Geometry: final body of the model. Coordinates: model frame, mm. Give positions to 0.01 mm unless a question says otherwise; leave off trailing zeros. Order: outer loops, then holes, each group sorted by start corner. A loop starts at its lowest first (then second) coordinate and runs counter-clockwise, first axis right, second up. Notation, with made-up numbers: (84.5, -25.75) -> (115.5, -25.75) arc R31 cw to (115.5, 4.25) -> close; hole circle Ø7 at (32, 89). An arc over 180 degrees is marked (long way). One line per item, written item: value. Start each with the question number.
```python
from build123d import *

# Parameters (mm, degrees)
SKETCH1_R           = 85.725
BOSS_EXTRUDE1_DEPTH = 6.35
CUT_EXTRUDE1_REACH  = 123.4
SKETCH2_R           = 1.5875
CUT_EXTRUDE2_REACH  = 123.4
SKETCH3_R           = 5
SKETCH3_R_2         = 3.175
CUT_EXTRUDE3_REACH  = 123.4
SKETCH5_R           = 1.4732
CENTER_HOLE_REACH   = 123.4
SKETCH6_R           = 5.0165


with BuildPart() as part:
    # Sketch1 → Boss-Extrude1 (new body)
    with BuildSketch(Plane(origin=(0, 0, 0), x_dir=(1, 0, 0), z_dir=(0, 1, 0))):
        with Locations(Location((0, 0, 0), (0, 0, 270))):
            Circle(SKETCH1_R)
    extrude(amount=BOSS_EXTRUDE1_DEPTH)

    # Sketch2 → Cut-Extrude1 (cut, up to next)
    with BuildSketch(Plane(origin=(0, 6.35, 0), x_dir=(1, 0, 0), z_dir=(0, 1, 0)), mode=Mode.PRIVATE) as cut_extrude1_sk1:
        with Locations(Location((-63.5, 44.45, 0), (0, 0, 270))):
            Circle(SKETCH2_R)
    cut_extrude1_tool1 = extrude(cut_extrude1_sk1.sketch, amount=-CUT_EXTRUDE1_REACH, mode=Mode.PRIVATE) & part.part
    # Sketch2 → Cut-Extrude1 (cut, up to next)
    with BuildSketch(Plane(origin=(0, 6.35, 0), x_dir=(1, 0, 0), z_dir=(0, 1, 0)), mode=Mode.PRIVATE) as cut_extrude1_sk2:
        with Locations(Location((63.5, 44.45, 0), (0, 0, 270))):
            Circle(SKETCH2_R)
    cut_extrude1_tool2 = extrude(cut_extrude1_sk2.sketch, amount=-CUT_EXTRUDE1_REACH, mode=Mode.PRIVATE) & part.part
    # Sketch2 → Cut-Extrude1 (cut, up to next)
    with BuildSketch(Plane(origin=(0, 6.35, 0), x_dir=(1, 0, 0), z_dir=(0, 1, 0)), mode=Mode.PRIVATE) as cut_extrude1_sk3:
        with Locations(Location((-63.5, -44.45, 0), (0, 0, 270))):
            Circle(SKETCH2_R)
    cut_extrude1_tool3 = extrude(cut_extrude1_sk3.sketch, amount=-CUT_EXTRUDE1_REACH, mode=Mode.PRIVATE) & part.part
    # Sketch2 → Cut-Extrude1 (cut, up to next)
    with BuildSketch(Plane(origin=(0, 6.35, 0), x_dir=(1, 0, 0), z_dir=(0, 1, 0)), mode=Mode.PRIVATE) as cut_extrude1_sk4:
        with Locations(Location((63.5, -44.45, 0), (0, 0, 270))):
            Circle(SKETCH2_R)
    cut_extrude1_tool4 = extrude(cut_extrude1_sk4.sketch, amount=-CUT_EXTRUDE1_REACH, mode=Mode.PRIVATE) & part.part
    add(cut_extrude1_tool1.solids().sort_by_distance((-63.5, 6.35, -44.45))[0], mode=Mode.SUBTRACT)
    add(cut_extrude1_tool2.solids().sort_by_distance((63.5, 6.35, -44.45))[0], mode=Mode.SUBTRACT)
    add(cut_extrude1_tool3.solids().sort_by_distance((-63.5, 6.35, 44.45))[0], mode=Mode.SUBTRACT)
    add(cut_extrude1_tool4.solids().sort_by_distance((63.5, 6.35, 44.45))[0], mode=Mode.SUBTRACT)

    # Sketch3 → Cut-Extrude2 (cut, up to next)
    with BuildSketch(Plane(origin=(0, 6.35, 0), x_dir=(1, 0, 0), z_dir=(0, 1, 0)), mode=Mode.PRIVATE) as cut_extrude2_sk1:
        with Locations(Location((38.522765446, -22.241129, 0), (0, 0, 270))):
            Circle(SKETCH3_R)
    cut_extrude2_tool1 = extrude(cut_extrude2_sk1.sketch, amount=-CUT_EXTRUDE2_REACH, mode=Mode.PRIVATE) & part.part
    # Sketch3 → Cut-Extrude2 (cut, up to next)
    with BuildSketch(Plane(origin=(0, 6.35, 0), x_dir=(1, 0, 0), z_dir=(0, 1, 0)), mode=Mode.PRIVATE) as cut_extrude2_sk2:
        with Locations(Location((0, 44.482258, 0), (0, 0, 270))):
            Circle(SKETCH3_R_2)
    cut_extrude2_tool2 = extrude(cut_extrude2_sk2.sketch, amount=-CUT_EXTRUDE2_REACH, mode=Mode.PRIVATE) & part.part
    # Sketch3 → Cut-Extrude2 (cut, up to next)
    with BuildSketch(Plane(origin=(0, 6.35, 0), x_dir=(1, 0, 0), z_dir=(0, 1, 0)), mode=Mode.PRIVATE) as cut_extrude2_sk3:
        with Locations(Location((-38.522765446, -22.241129, 0), (0, 0, 270))):
            Circle(SKETCH3_R)
    cut_extrude2_tool3 = extrude(cut_extrude2_sk3.sketch, amount=-CUT_EXTRUDE2_REACH, mode=Mode.PRIVATE) & part.part
    add(cut_extrude2_tool1.solids().sort_by_distance((38.522765, 6.35, 22.241129))[0], mode=Mode.SUBTRACT)
    add(cut_extrude2_tool2.solids().sort_by_distance((0, 6.35, -44.482258))[0], mode=Mode.SUBTRACT)
    add(cut_extrude2_tool3.solids().sort_by_distance((-38.522765, 6.35, 22.241129))[0], mode=Mode.SUBTRACT)

    # Sketch5 → Cut-Extrude3 (cut, up to next)
    with BuildSketch(Plane(origin=(0, 6.35, 0), x_dir=(1, 0, 0), z_dir=(0, 1, 0)), mode=Mode.PRIVATE) as cut_extrude3_sk1:
        with Locations(Location((-15.50035, 59.982608, 0), (0, 0, 270))):
            Circle(SKETCH5_R)
    cut_extrude3_tool1 = extrude(cut_extrude3_sk1.sketch, amount=-CUT_EXTRUDE3_REACH, mode=Mode.PRIVATE) & part.part
    # Sketch5 → Cut-Extrude3 (cut, up to next)
    with BuildSketch(Plane(origin=(0, 6.35, 0), x_dir=(1, 0, 0), z_dir=(0, 1, 0)), mode=Mode.PRIVATE) as cut_extrude3_sk2:
        with Locations(Location((15.50035, 59.982608, 0), (0, 0, 270))):
            Circle(SKETCH5_R)
    cut_extrude3_tool2 = extrude(cut_extrude3_sk2.sketch, amount=-CUT_EXTRUDE3_REACH, mode=Mode.PRIVATE) & part.part
    # Sketch5 → Cut-Extrude3 (cut, up to next)
    with BuildSketch(Plane(origin=(0, 6.35, 0), x_dir=(1, 0, 0), z_dir=(0, 1, 0)), mode=Mode.PRIVATE) as cut_extrude3_sk3:
        with Locations(Location((-15.50035, 28.981908, 0), (0, 0, 270))):
            Circle(SKETCH5_R)
    cut_extrude3_tool3 = extrude(cut_extrude3_sk3.sketch, amount=-CUT_EXTRUDE3_REACH, mode=Mode.PRIVATE) & part.part
    # Sketch5 → Cut-Extrude3 (cut, up to next)
    with BuildSketch(Plane(origin=(0, 6.35, 0), x_dir=(1, 0, 0), z_dir=(0, 1, 0)), mode=Mode.PRIVATE) as cut_extrude3_sk4:
        with Locations(Location((15.50035, 28.981908, 0), (0, 0, 270))):
            Circle(SKETCH5_R)
    cut_extrude3_tool4 = extrude(cut_extrude3_sk4.sketch, amount=-CUT_EXTRUDE3_REACH, mode=Mode.PRIVATE) & part.part
    add(cut_extrude3_tool1.solids().sort_by_distance((-15.50035, 6.35, -59.982608))[0], mode=Mode.SUBTRACT)
    add(cut_extrude3_tool2.solids().sort_by_distance((15.50035, 6.35, -59.982608))[0], mode=Mode.SUBTRACT)
    add(cut_extrude3_tool3.solids().sort_by_distance((-15.50035, 6.35, -28.981908))[0], mode=Mode.SUBTRACT)
    add(cut_extrude3_tool4.solids().sort_by_distance((15.50035, 6.35, -28.981908))[0], mode=Mode.SUBTRACT)

    # Sketch6 → center_hole (cut, up to next)
    with BuildSketch(Plane(origin=(0, 6.35, 0), x_dir=(1, 0, 0), z_dir=(0, 1, 0)), mode=Mode.PRIVATE) as center_hole_sk1:
        with Locations(Location((0, 0, 0), (0, 0, 270))):
            Circle(SKETCH6_R)
    center_hole_tool1 = extrude(center_hole_sk1.sketch, amount=-CENTER_HOLE_REACH, mode=Mode.PRIVATE) & part.part
    add(center_hole_tool1.solids().sort_by_distance((0, 6.35, 0))[0], mode=Mode.SUBTRACT)


solid = part.part
```
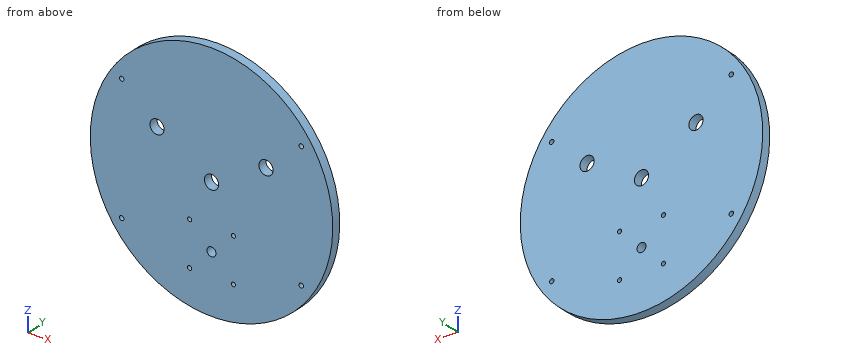
1. Cut plane D-D, the plane x = 70.5. Return loops of the section in (y, z).
2. Cut plane C-C, the plane y = 4.5. State how many separate pieces and enclosed holes the cut face has, then the cut area to 3 significant figures.
3. Cut plane B-B, the plane x = -36.5. Return loops of the section in (y, z), then the cut area to 3 significant figures.
4. Pin query (flat end, axial travel): P1, Ø2.5, axis at x = -15.5, z = -28.98, coming from the -Y side; P2, Ø2, axis at y = 4, z = 17, coming from the -X side; P3, Ø1, axis at y = 2.5, z = 45, coming from the -X side; P4, Ø1, axis at y = 0.5, z = 5.5, coming from the -X side. Return the tip coordinate at first contact, or that it passes through.
5. Material intervals for L1, parallel to X at y = 2.25, z = 45; L2, parallel to Z at x = -64, y = 4; L3, parallel to Z at x = -16.5, y = 5, sorted ascending. Write a range as [from, to].
Answers follow:
1. outline: (0, -48.77) -> (6.35, -48.77) -> (6.35, 48.77) -> (0, 48.77) -> close
2. separate pieces: 1
2. enclosed holes: 12
2. area: 22,800 mm²
3. outline: (0, -77.57) -> (6.35, -77.57) -> (6.35, 17.67) -> (0, 17.67) -> close; (0, 26.81) -> (6.35, 26.81) -> (6.35, 77.57) -> (0, 77.57) -> close
3. area: 927 mm²
4. P1: passes through
4. P2: stops at x = -84.22
4. P3: stops at x = -73.27
4. P4: stops at x = -85.58
5. L1: x = [-72.96, -64.99], [-62.01, 62.01], [64.99, 72.96]
5. L2: z = [-57.03, -45.96], [-42.94, 42.94], [45.96, 57.03]
5. L3: z = [-84.12, -61.06], [-58.9, -30.06], [-27.9, 84.12]
